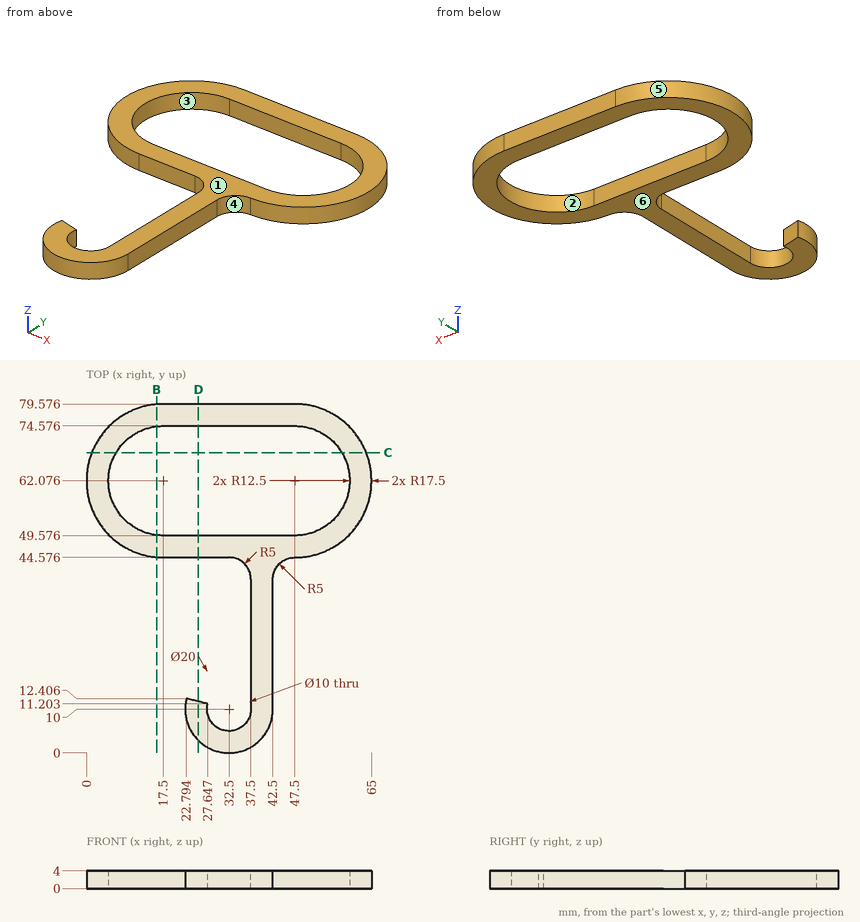
Design review of the part shown in the three views and the two pictorial views. Dimensions are in mm from the part's minimum x, y and z. A direction names the side the tool comes from. Round coordinates to 2 decimals unless told otherwise and drop trailing zeros. Write each loop counter-clockwise with the first axis right and the second up, starting at its lowest first coordinate (ties: lowest second). Pieces come first, ordered by that corner, then holes. Notation, with made-up numbers: (70, 62.25) - (106, 62.25) arc R13 cw to (106, 80.25) - close; hole circle Ø3 at (56, 38.5). An arc over 180 degrees is marked (long way). Return JSON: item names as keys, results as strings. Group by question number.
Item 1: We need section C-C on y = 68.5. Write out the cut boundary in (x, z).
Item 2: The part is to be moulded in two halves that separate along Y. For the marked faces 3, 4, 5 and 6, say which applies: pulls with the +Y half, pulls with the -Y half, needs draft (parallel to the pull), parting line crosses it, or undercut.
Item 3: We need section D-D on x = 25.5. Write out the cut boundary in (y, z) (1 decimal).
Item 4: Insertion check: P1, Ø1.2, axis at y = 23.5, z = 2.5, coming from the -X side; P2, Ø8, axis at x = 58.5, y = 60.5, coming from the -Z side; P3, Ø6, axis at x = 45, y = 69, coming from the +Z side; P4, Ø1, axis at x = 24.5, z = 1, coming from the -Y side (1 decimal). Each pin has a flat end and moves straight along its axis. Give the tip position at first contact, or say it passes through.
Item 5: We need section B-B on x = 16. Write out the cut boundary in (y, z) (1 decimal).
Item 6: Machinability: for the marked faces 1 and 2, which of the approach directions +Z, -Z, +X, -X, +Y, -Y give a long, thin tool a straight path to every point of the face, cutting with its end or side? Answer none if there is none.
Item 7: For probe 1 along Y at (x, z) = (32.5, 1.95); probe 2 along X at (y, z) = (10, 1.65); probe 3 along Y at (x, z) = (26.5, 0.8) (1 decimal), list the stretches that pass through material, from the lowest coordinate up. Write a range as [from, to].
Model answer:
{
 "1": {"outline": "(1.22, 0) - (6.78, 0) - (6.78, 4) - (1.22, 4) - close; (58.22, 0) - (63.78, 0) - (63.78, 4) - (58.22, 4) - close"},
 "2": {"face 3": "undercut", "face 4": "pulls with the -Y half", "face 5": "parting line crosses it", "face 6": "needs draft"},
 "3": {"outline": "(2.9, 0) - (11.7, 0) - (11.7, 4) - (2.9, 4) - close; (44.6, 0) - (49.6, 0) - (49.6, 4) - (44.6, 4) - close; (74.6, 0) - (79.6, 0) - (79.6, 4) - (74.6, 4) - close"},
 "4": {"P1": "stops at x = 37.5", "P2": "stops at z = 0", "P3": "passes through", "P4": "stops at y = 3.4"},
 "5": {"outline": "(44.6, 0) - (49.7, 0) - (49.7, 4) - (44.6, 4) - close; (74.5, 0) - (79.5, 0) - (79.5, 4) - (74.5, 4) - close"},
 "6": {"face 1": "+Z, +X, -X, +Y, -Y", "face 2": "+Z, -Z"},
 "7": {"probe 1": "y = [0, 5], [44.58, 49.58], [74.58, 79.58]", "probe 2": "x = [22.5, 27.5], [37.5, 42.5]", "probe 3": "y = [2, 11.5], [44.6, 49.6], [74.6, 79.6]"}
}
